```python
from build123d import *

# Parameters (mm, degrees)
RESSALTO_EXTRUS_O1_DEPTH = 3
ESBO_O3_W                = 3
ESBO_O3_H                = 1.25
RESSALTO_EXTRUS_O2_DEPTH = 2
ESBO_O4_W                = 3
ESBO_O4_H                = 1.25
RESSALTO_EXTRUS_O3_DEPTH = 2


with BuildPart() as part:
    # Esboço1 → Ressalto-extrusão1 (new body)
    with BuildSketch(Plane(origin=(0, 0, 0), x_dir=(1, 0, 0), z_dir=(0, 1, 0))):
        Polygon((0, -28), (0, -2), (32, -2), (32, 0), (0, 0), (0, 26.5), (-2, 26.5), (-2, -30), (32, -30), (32, -28), align=None)
    extrude(amount=RESSALTO_EXTRUS_O1_DEPTH)

    # Esboço3 → Ressalto-extrusão2 (add)
    with BuildSketch(Plane.ZY.offset(2)):
        with Locations((-13.75, -0.625)):
            Rectangle(ESBO_O3_W, ESBO_O3_H)
        with Locations((17.25, -0.625)):
            Rectangle(ESBO_O3_W, ESBO_O3_H)
    extrude(amount=-RESSALTO_EXTRUS_O2_DEPTH)

    # Esboço4 → Ressalto-extrusão3 (add)
    with BuildSketch(Plane.XY.offset(30)):
        with Locations((15, -0.625)):
            Rectangle(ESBO_O4_W, ESBO_O4_H)
    ressalto_extrus_o3 = extrude(amount=-RESSALTO_EXTRUS_O3_DEPTH)

    # Espelhar1: Ressalto-extrusão3 across plane
    add(ressalto_extrus_o3.mirror(Plane.XY.offset(15)))


solid = part.part
```
Geometry: final body of the model. Coordinates: model frame, mm. A direction names the side the tool comes from. Give positions to 0.01 mm unless a question says otherwise; leave off trailing zeros. Write each loop counter-clockwise with the first axis right and the second up, starting at its lowest first coordinate (ties: lowest second). Pieces come first, ordered by that corner, then holes.
1. Line query: probe 1 along Z at (x, y) = (30, 0.5); probe 2 along X at (y, z) = (1.2, 27.5); probe 3 along Y at (x, z) = (7, 1). Output: solid intervals per line, ascending.
2. Reachability of faces 1 (the flat face through (-1, 0, -21)), 2 (the flat face through (-1, -1, 15.75)), 3 (the flat face through (0, 1, 15)), 4 (the flat face through (24, 0, 1)) from +Z, -Z, +X, -X, +Y, -Y: full face, straight path, thin tool, end or side. Return the list, or none.
3. Pin query (flat end, axial travel): P1, Ø1.6, axis at x = 20.5, z = 28.5, coming from the -Y side; P2, Ø0.6, axis at y = -1, z = 1.5, coming from the -X side; P3, Ø2, axis at y = 0.5, z = -15, coming from the +X side. Return the tip coordinate at first contact, or that it passes through.
4. Section query C-C, the plane y = 2.4. Return loops of the section in (x, z).
5. Section query A-A, the plane y = -0.7. Return loops of the section in (x, z), then the cut area to 3 significant figures.
6. Draft query along Z for faces 5 (the flat face through (15, 1, 30)), 6 (the flat face through (-1, -1, -12.25)), 7 (the flat face through (0, 1, -13)). Return one class per face: released by +Z, released by -Z, zero draft, split by the parting line, or undercut.
7. Section query B-B, the plane x = 27. Return loops of the section in (y, z).
8. Section query D-D, the plane z = -13. Return loops of the section in (x, y).
Computed:
1. probe 1: z = 0 to 2, 28 to 30
1. probe 2: x = -2 to 0
1. probe 3: y = 0 to 3
2. face 1: -Z, +X, -X, -Y
2. face 2: +X, -X, -Y
2. face 3: +X, +Y, -Y
2. face 4: +Z, -Z, +X, -Y
3. P1: stops at y = 0
3. P2: stops at x = 13.5
3. P3: stops at x = 0
4. outline: (-2, -26.5) - (0, -26.5) - (0, 0) - (32, 0) - (32, 2) - (0, 2) - (0, 28) - (32, 28) - (32, 30) - (-2, 30) - close
5. outline: (-2, -15.25) - (0, -15.25) - (0, -12.25) - (-2, -12.25) - close; (-2, 15.75) - (0, 15.75) - (0, 18.75) - (-2, 18.75) - close; (13.5, 0) - (16.5, 0) - (16.5, 2) - (13.5, 2) - close; (13.5, 28) - (16.5, 28) - (16.5, 30) - (13.5, 30) - close
5. area: 24.0 mm2
6. face 5: released by +Z
6. face 6: undercut
6. face 7: zero draft
7. outline: (0, 0) - (3, 0) - (3, 2) - (0, 2) - close; (0, 28) - (3, 28) - (3, 30) - (0, 30) - close
8. outline: (-2, -1.25) - (0, -1.25) - (0, 3) - (-2, 3) - close
